Autodesk Inventor part; units mm, degrees
ref_plane "YZ Plane" through (0, 0, 0) normal (1, 0, 0) x (0, 1, 0)
ref_plane "XZ Plane" through (0, 0, 0) normal (0, 1, 0) x (-1, 0, 0)
ref_plane "XY Plane" through (0, 0, 0) normal (0, 0, 1) x (1, 0, 0)
sketch "Sketch1" plane through (0, 0, 0) normal (0, 0, 1) x (1, 0, 0)
  line L0 (0, 0) -> (55, 0)
  line L1 (55, 0) -> (55, 30)
  line L2 (55, 30) -> (50, 30)
  line L3 (50, 30) -> (50, 5)
  line L4 (50, 5) -> (5, 5)
  line L5 (5, 5) -> (5, 30)
  line L6 (5, 30) -> (0, 30)
  line L7 (0, 30) -> (0, 0)
  dimension "d0" = 55
  dimension "d1" = 30
  dimension "d2" = 5
  dimension "d3" = 25
  dimension "d4" = 45
  dimension "d5" = 25
  dimension "d6" = 5
extrude "Extrusion1" add sketch "Sketch1" along normal blind 25
sketch "Sketch2" plane through (55, 0, 0) normal (1, 0, 0) x (0, 0, -1)
  circle A0 centre (-12.5, 20) radius 2.5
  line L0 (0, 30) -> (-25, 30)
  line L1 (0, 0) -> (0, 30)
  dimension "d9" = 5
  dimension "d10" = 10
  dimension "d11" = 12.5
extrude "Extrusion2" cut sketch "Sketch2" against normal through all
sketch "Sketch3" plane through (5, 5, 0) normal (0, 1, 0) x (1, 0, 0)
  line L0 (12.5, -6.5) -> (32.5, -6.5)
  line L1 (32.5, -6.5) -> (32.5, -18.5)
  line L2 (32.5, -18.5) -> (12.5, -18.5)
  line L3 (12.5, -18.5) -> (12.5, -6.5)
  line L4 (12.5, -6.5) -> (32.5, -18.5) construction
  line L5 (32.5, -6.5) -> (12.5, -18.5) construction
  line L6 (45, 0) -> (0, 0)
  line L7 (0, 0) -> (0, -25)
  point P0 (-5, 0)
  point P1 (22.5, -12.5)
  dimension "d14" = 20
  dimension "d15" = 12
  dimension "d16" = 12.5
  dimension "d17" = 22.5
extrude "Extrusion3" cut sketch "Sketch3" against normal through all
sketch "Sketch4" plane through (5, 5, 0) normal (0, 1, 0) x (1, 0, 0)
  circle A0 centre (5.25, -12.5) radius 3.625
  circle A1 centre (39.75, -12.5) radius 3.625
  line L0 (0, -10) -> (0, -15)
  line L1 (45, 0) -> (45, -25)
  line L2 (45, -25) -> (0, -25)
  point P0 (-5, 0)
  dimension "d20" = 7.25
  dimension "d21" = 7.25
  dimension "d22" = 5.25
  dimension "d23" = 5.25
  dimension "d24" = 12.5
  dimension "d25" = 12.5
extrude "Extrusion4" cut sketch "Sketch4" against normal blind 2.1735 draft -45
sketch "Sketch5" plane through (10.25, 2.8265, 12.5) normal (0, 1, 0) x (1, 0, 0)
  circle A0 centre (0, 0) radius 1.4515
  circle A1 centre (34.5, 0) radius 1.4515
  line L0 (39.75, 12.5) -> (39.75, -12.5)
  point P0 (-10.25, 12.5)
  dimension "d28" = 2.903
  dimension "d29" = 2.903
  dimension "d30" = 5.25
extrude "Extrusion5" cut sketch "Sketch5" against normal through all
properties part number "2nd to 3rd arm linking clamp"
Build history of the part. All positions in model axes, mm. A direction names the side the tool comes from. Give positions to 0.01 mm unless a question says otherwise; leave off trailing zeros. Order: outer loops, then holes, each group sorted by start corner. A loop starts at its lowest first (then second) coordinate and runs counter-clockwise, first axis right, second up. Notation, with made-up numbers: M 88.5,-11.75 L 120.5,-11.75 A20 cw 120.5,22.25 Z; hole C 10,43 d1. An arc over 180 degrees is marked long. Put each result on its own line as item: value.
Item 1: Slice it at C-C, the plane z = 12.5. Give the number of separate pieces and of enclosed holes in the cut face, plus the area to 3 significant figures.
From the geometry:
separate pieces: 6
enclosed holes: 0
area: 337 mm2
Item 2: Two-plate mould, pull along Z, no slides. Class faces 1 (the flat face through (50, 15, 12)), 2 (the flat face through (27, 4, 25)), 3 (the flat face through (27, 3, 6.5)): +Z half, -Z half, draft (parallel to the pull), parting line (faces both ways), or undercut.
From the geometry:
face 1: draft
face 2: +Z half
face 3: undercut
Item 3: Slice it at D-D, the plane x = 29. Write the cut outline in (y, z).
From the geometry:
outline: M 0,0 L 5,0 L 5,6.5 L 0,6.5 Z; M 0,18.5 L 5,18.5 L 5,25 L 0,25 Z
Item 4: Slice it at A-A, the plane z = 7.5. Write the cut outline in (x, y).
From the geometry:
outline: M 0,0 L 17.5,0 L 17.5,5 L 5,5 L 5,30 L 0,30 Z; M 37.5,0 L 55,0 L 55,30 L 50,30 L 50,5 L 37.5,5 Z
Item 5: 3-axis set-ups, long thin cutter, end or side, ignore diameter. For faces 4 (the flat face through (28, 5, 4)), 5 (the flat face through (17.5, 3, 13)), 6 (the flat face through (0, 15, 12)): which of +Z, -Z, +X, -X, +Y, -Y reach the whole face in a straight line?
From the geometry:
face 4: +Z, -Z, +Y
face 5: +Y, -Y
face 6: +Z, -Z, -X, +Y, -Y
Item 6: Probe line 1 (X direction, y = 2, z = 12.5); line 2 (X direction, y = 15, z = 13.25); line 3 (Z direction, x = 44.75, y = 1.1). List the from-to ranges inside material, lowest first. Write a range as [from, to].
From the geometry:
line 1: x = [0, 8.8], [11.7, 17.5], [37.5, 43.3], [46.2, 55]
line 2: x = [0, 5], [50, 55]
line 3: z = [0, 11.05], [13.95, 25]
Item 7: Slice it at B-B, the plane y = 25.5. Write the cut outline in (x, z).
From the geometry:
outline: M 0,0 L 5,0 L 5,25 L 0,25 Z; M 50,0 L 55,0 L 55,25 L 50,25 Z
Item 8: Flat gauge pin, fed straight in: pin 1 Ø7.5 at (x, z) = (35, 9.5) entering from +Y. Where does the tip first touch, or does it go through?
From the geometry:
pin 1: stops at y = 5
